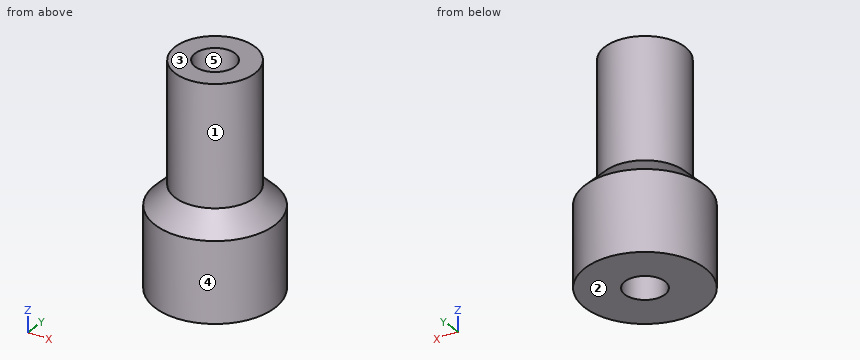
```python
from build123d import *

# Parameters (mm, degrees)
BASE_SKETCH_R           = 3
BASE_SKETCH_R_2         = 2
EXTRUDE_PIN_THICK_DEPTH = 4
BASE_SKETCH_3_R         = 2
BASE_SKETCH_3_R_2       = 1
EXTRUDE_PIN_THIN_DEPTH  = 11
CHAMFER_2_SIZE          = 1


with BuildPart() as part:
    # Base Sketch → Extrude Pin Thick (new body)
    with BuildSketch(Plane.XY):
        Circle(BASE_SKETCH_R)
        Circle(BASE_SKETCH_R_2, mode=Mode.SUBTRACT)
    extrude(amount=EXTRUDE_PIN_THICK_DEPTH)

    # Base Sketch<3> → Extrude Pin Thin (add)
    with BuildSketch(Plane.XY):
        Circle(BASE_SKETCH_3_R)
        Circle(BASE_SKETCH_3_R_2, mode=Mode.SUBTRACT)
    extrude(amount=EXTRUDE_PIN_THIN_DEPTH)

    # Chamfer 2
    chamfer_2_edges = [part.edges().sort_by_distance(p)[0] for p in [
        (-2, 0, 4),
    ]]
    chamfer(chamfer_2_edges, length=CHAMFER_2_SIZE - 0.0001)  # a hair under: the kernel refuses the full size


solid = part.part
```
Work out the finished part from the listing and answer in its coordinate system (mm). Face numbers are marked on the shaded views. A direction names the side the tool comes from. Round coordinates to 2 decimals unless told otherwise and drop trailing zeros. Order: outer loops, then holes, each group sorted by start corner. A loop starts at its lowest first (then second) coordinate and runs counter-clockwise, first axis right, second up.
Q1. A tool of negligible diameter and unlimited length cuts with its end or side. For the marked faces 1 and 2, from which of +Z, -Z, +X, -X, +Y, -Y can it reach the whole face along a straight path? Write none if from no direction.
Solution:
face 1: +Z
face 2: -Z, +X, -X, +Y, -Y
Q2. The mould has two halves that part along Y. Classify the marked faces 3, 4 and 5: pulls with the +Y half, pulls with the -Y half, needs draft (parallel to the pull), parting line crosses it, or undercut.
Solution:
face 3: needs draft
face 4: parting line crosses it
face 5: undercut
Q3. A cutting plane is placed at C-C, the plane z = 2.25. Determine the outline of the cut face in (x, y).
Solution:
outline: circle Ø6 at (0, 0); hole circle Ø2 at (0, 0)
Q4. Given pin 1 Ø2 at (y, z) = (-0.5, 6.5) entering from +X; pin 2 Ø3 at (y, z) = (-0.5, 6) entering from +X, each flat-ended and moving along its own axis, determine where each tip first touches the part or whether it passes through.
Solution:
pin 1: stops at x = 2
pin 2: stops at x = 2.47
Q5. A cutting plane is placed at D-D, the plane z = 6.5. Determine the outline of the cut face in (x, y), then the cut area to 3 significant figures.
Solution:
outline: circle Ø4 at (0, 0); hole circle Ø2 at (0, 0)
area: 9.42 mm2
Q6. Find the intervals of material crossed by line 1 along Y through (x, z) = (0, 5.5); line 2 along Y through (x, z) = (0, 3); line 3 along X through (y, z) = (0.45, 6.5), in increasing order.
Solution:
line 1: y = -2 to -1, 1 to 2
line 2: y = -3 to -1, 1 to 3
line 3: x = -1.95 to -0.89, 0.89 to 1.95
